Autodesk Inventor part; units mm, degrees
ref_plane "YZ Plane" through (0, 0, 0) normal (1, 0, 0) x (0, 1, 0)
ref_plane "XZ Plane" through (0, 0, 0) normal (0, 1, 0) x (-1, 0, 0)
ref_plane "XY Plane" through (0, 0, 0) normal (0, 0, 1) x (1, 0, 0)
sketch "Sketch1" plane through (0, 0, 0) normal (0, 0, 1) x (1, 0, 0)
  line L0 (-395.4763, 28.0534) -> (214.1237, 28.0534)
  line L1 (214.1237, 28.0534) -> (214.1237, -124.3466)
  line L2 (214.1237, -124.3466) -> (-395.4763, -124.3466)
  line L3 (-395.4763, -124.3466) -> (-395.4763, 28.0534)
  line L4 (100.4888, 124.4295) -> (100.4888, 286.3545)
  line L5 (100.4888, 286.3545) -> (135.4138, 286.3545)
  line L6 (137.9237, 286.3545) -> (137.9237, 124.4295)
  line L7 (137.9237, 124.4295) -> (100.4888, 124.4295)
  point P0 (0, 0)
  dimension "d0" = 609.6
  dimension "d1" = 152.4
  dimension "d7" = 161.925
  dimension "d8" = 34.925
extrude "Extrusion1" add sketch "Sketch1" along normal blind 152.4
sketch "Sketch4" plane through (214.1237, -124.3466, 0) normal (1, 0, 0) x (0, 0, -1)
  circle A0 centre (-76.2, 76.2) radius 5.1594
  line L0 (-152.4, 0) -> (-152.4, 152.4)
  line L1 (0, 152.4) -> (-152.4, 152.4)
  point P0 (0, 124.3466)
  dimension "d1" = 152.4
  dimension "d9" = 10.3187
extrude "Extrusion2" cut sketch "Sketch4" against normal blind 609.6
sketch "Sketch5" plane through (-395.4763, 28.0534, 0) normal (0, 1, 0) x (1, 0, 0)
  line L0 (609.6, -152.4) -> (0, -152.4)
  line L1 (0, -152.4) -> (0, 0)
  line L2 (0, 0) -> (609.6, 0)
  line L3 (609.6, 0) -> (609.6, -152.4)
  line L4 (609.6, -152.4) -> (0, -152.4)
  line L5 (609.6, 0) -> (609.6, -152.4)
  line L6 (0, 0) -> (0, -152.4)
  line L7 (0, 0) -> (609.6, 0)
  line L8 (297.18, -104.775) -> (312.42, -104.775)
  line L9 (312.42, -104.775) -> (312.42, -47.625)
  line L10 (312.42, -47.625) -> (297.18, -47.625)
  line L11 (297.18, -47.625) -> (297.18, -104.775)
  line L12 (297.18, -104.775) -> (312.42, -47.625) construction
  line L13 (312.42, -104.775) -> (297.18, -47.625) construction
  point P0 (395.4763, 0)
  point P1 (297.0135, -78.1466)
  point P2 (312.2535, -78.0634)
  point P3 (312.2535, -74.3366)
  point P4 (304.8, -76.2)
  dimension "d1" = 152.4
  dimension "d48" = 15.24
  dimension "d49" = 57.15
  dimension "d50" = 47.625
  dimension "d51" = 47.625
extrude "Extrusion3" cut sketch "Sketch5" against normal blind 609.6 contours L11 L10 L9 L8
fillet "Fillet1" radius 6.35 4 edges at (-90.6763, 28.0534, 47.625) (-90.6763, 28.0534, 104.775) (-90.6763, -124.3466, 47.625) (-90.6763, -124.3466, 104.775)
chamfer "Chamfer1" distance 3.175 angle 45 1 edges at (214.1237, -48.1466, 81.3594) measured on face at (16.0037, -48.5618, 71.0574)
chamfer "Chamfer2" distance 3.175 angle 45 1 edges at (-395.4763, -48.1466, 81.3594) measured on face at (-296.4163, -48.5618, 71.0574)
sketch "Sketch6" plane through (-395.4763, 28.0534, 0) normal (0, 1, 0) x (1, 0, 0)
  line L0 (609.6, 0) -> (609.6, -152.4)
  line L1 (609.6, -152.4) -> (0, -152.4)
  line L2 (0, -152.4) -> (0, 0)
  line L3 (0, 0) -> (609.6, 0)
  line L4 (609.6, -84.5344) -> (609.6, -67.8656)
  line L5 (609.6, -76.2) -> (625.475, -76.2) construction
  circle A0 centre (593.725, -76.2) radius 3.175
  line L6 (0, 0) -> (0, -152.4)
  circle A1 centre (15.875, -76.2) radius 3.175
  line L7 (297.18, -41.275) -> (312.42, -41.275)
  line L8 (312.42, -111.125) -> (312.42, -41.275)
  line L9 (312.42, -111.125) -> (297.18, -111.125)
  line L10 (297.18, -41.275) -> (297.18, -111.125)
  point P0 (395.4763, 0)
  dimension "d1" = 152.4
  dimension "d30" = 6.35
  dimension "d34" = 6.35
extrude "Extrusion4" cut sketch "Sketch6" against normal blind 101.6 contours A0 | A1
sketch "Sketch7" plane through (-395.4763, 28.0534, 0) normal (0, 1, 0) x (1, 0, 0)
  circle A0 centre (593.725, -76.2) radius 3.175 construction
  circle A1 centre (15.875, -76.2) radius 3.175
  line L0 (609.6, 0) -> (609.6, -152.4) construction
  line L1 (609.6, -152.4) -> (0, -152.4)
  line L2 (0, -152.4) -> (0, 0)
  line L3 (0, 0) -> (609.6, 0)
  line L4 (609.6, -152.4) -> (0, -152.4)
  line L5 (565.15, -152.4) -> (565.15, 0) construction
  line L6 (609.6, 0) -> (609.6, -152.4) construction
  line L7 (297.18, -41.275) -> (312.42, -41.275)
  line L8 (312.42, -111.125) -> (312.42, -41.275)
  line L9 (312.42, -111.125) -> (297.18, -111.125)
  line L10 (297.18, -41.275) -> (297.18, -111.125)
  line L11 (609.6, -76.2) -> (629.3437, -76.2) construction
  line L12 (629.3437, -56.1975) -> (609.6, -56.1975) construction
  line L13 (629.3437, -96.2025) -> (609.6, -96.2025) construction
  line L14 (609.6, -96.2025) -> (529.5756, -96.2025) construction
  line L15 (609.6, -56.1975) -> (531.5543, -56.1975) construction
  circle A2 centre (565.15, -96.2025) radius 3.175
  circle A3 centre (565.15, -56.1975) radius 3.175
  point P0 (395.4763, 0)
  dimension "d1" = 152.4
  dimension "d37" = 44.45
  dimension "d85" = 20.0025
  dimension "d86" = 40.005
  dimension "d87" = 6.35
  dimension "d88" = 6.35
  dimension "d89" = 44.45
extrude "Extrusion5" cut sketch "Sketch7" against normal blind 28.575 contours A2 | A3
sketch "Sketch9" plane through (-395.4763, -124.3466, 0) normal (0, -1, 0) x (1, 0, 0)
  line L0 (609.6, 152.4) -> (609.6, 0)
  line L1 (609.6, 0) -> (0, 0)
  line L2 (0, 0) -> (0, 152.4)
  line L3 (0, 152.4) -> (609.6, 152.4)
  line L4 (312.42, 41.275) -> (297.18, 41.275)
  line L5 (297.18, 111.125) -> (297.18, 41.275)
  line L6 (297.18, 111.125) -> (312.42, 111.125)
  line L7 (312.42, 41.275) -> (312.42, 111.125)
  line L8 (0, 76.2) -> (609.6, 76.2) construction
  circle A0 centre (218.44, 76.2) radius 19.685
  point P0 (395.4763, 0)
  dimension "d1" = 152.4
  dimension "d65" = 39.37
  dimension "d66" = 78.74
  dimension "d69" = 0
extrude "Extrusion8" cut sketch "Sketch9" against normal blind 63.5 contours A0
sketch "Sketch10" plane through (0, 0, 152.4) normal (0, 0, 1) x (1, 0, 0)
  line L0 (214.1237, 28.0534) -> (214.1237, -124.3466)
  line L1 (214.1237, -124.3466) -> (-395.4763, -124.3466)
  line L2 (-395.4763, -124.3466) -> (-395.4763, 28.0534)
  line L3 (-395.4763, 28.0534) -> (214.1237, 28.0534)
  line L4 (-157.3513, -124.3466) -> (-196.7213, -124.3466)
  line L5 (-157.3513, -60.8466) -> (-196.7213, -60.8466)
  line L6 (-157.3513, -124.3466) -> (-196.7213, -124.3466)
  line L7 (-157.3513, -92.075) -> (-196.7213, -92.075)
  line L8 (-177.0363, -92.075) -> (-177.0363, -60.8466)
  point P0 (0, 0)
  dimension "d1" = 152.4
  dimension "d72" = 31.2284
hole "Hole1" at (-177.0363, -92.075, 152.4) direction (0, 0, -1) diameter 3.9624 depth 13.6144 tip angle 118
sketch "Sketch11" plane through (214.1237, -124.3466, 0) normal (1, 0, 0) x (0, 0, -1)
  circle A0 centre (-76.2, 12.7) radius 3.175
  circle A1 centre (-76.2, 42.0133) radius 3.175
  point P0 (0, 124.3466)
  dimension "d1" = 152.4
extrude "Extrusion9" cut sketch "Sketch11" against normal blind 28.575
thread "Thread7"
thread "Thread8"
sketch "Sketch12" plane through (0, 0, 0) normal (0, 0, -1) x (-1, 0, 0)
  line L0 (-214.1237, -124.3466) -> (-214.1237, 28.0534) construction
  line L1 (-214.1237, 28.0534) -> (395.4763, 28.0534) construction
  line L2 (395.4763, 28.0534) -> (395.4763, -124.3466) construction
  line L3 (395.4763, -124.3466) -> (-214.1237, -124.3466) construction
  line L4 (90.6763, 28.0534) -> (90.6763, -124.3466) construction
  line L5 (392.3013, -42.9872) -> (392.3013, -53.306)
  line L6 (-36.3237, -111.6466) -> (90.6763, -111.6466) construction
  line L7 (90.6763, -111.6466) -> (90.6763, 15.3534) construction
  line L8 (90.6763, 15.3534) -> (-36.3237, 15.3534) construction
  line L9 (-36.3237, 15.3534) -> (-36.3237, -111.6466) construction
  line L10 (118.2888, 15.3534) -> (-69.9987, 15.3534) construction
  line L11 (118.2888, -10.0466) -> (-69.9987, -10.0466) construction
  line L12 (65.2763, 28.0534) -> (65.2763, -124.3466) construction
  circle A0 centre (65.2763, -10.0466) radius 4.7625
  circle A1 centre (-10.9237, -10.0466) radius 4.7625
  circle A2 centre (65.2763, -86.2466) radius 4.7625
  circle A3 centre (-10.9237, -86.2466) radius 4.7625
  line L13 (63.0639, -10.0466) -> (251.3514, -10.0466) construction
  line L14 (116.0763, 28.0534) -> (116.0763, -124.3466) construction
  circle A4 centre (116.0763, -10.0466) radius 4.7625
  circle A5 centre (192.2763, -10.0466) radius 4.7625
  circle A6 centre (116.0763, -86.2466) radius 4.7625
  circle A7 centre (192.2763, -86.2466) radius 4.7625
  point P0 (0, 0)
  point P1 (181.3527, 0)
  dimension "d1" = 152.4
  dimension "d97" = 127
  dimension "d98" = 127
  dimension "d99" = 25.4
  dimension "d100" = 25.4
  dimension "d101" = 9.525
  dimension "d104" = 76.2
  dimension "d107" = 76.2
extrude "Extrusion10" cut sketch "Sketch12" against normal through all
properties part number "block"
Work out the finished part from the listing and answer in its coordinate system (mm). A direction names the side the tool comes from. Give positions to 0.01 mm unless a question says otherwise; leave off trailing zeros. Answer as CSV lines item,"result".
Q1. Find the intervals of material crossed by probe 1 along Y at (x, z) = (205.25, 76.2); probe 2 along Y at (x, z) = (-190.5, 98); probe 3 along Y at (x, z) = (198, 76.2), in increasing order. Write a range as [from, to].
A:
probe 1,"y = [-124.35, -114.82], [-108.47, -85.51], [-79.16, -53.31], [-42.99, 28.05]"
probe 2,"y = [-124.35, -90.67], [-81.83, -14.47], [-5.63, 28.05]"
probe 3,"y = [-124.35, -114.82], [-108.47, -85.51], [-79.16, -73.55]"
Q2. A tool of negligible diameter and unlimited length cuts with its end or side. For faces 1 (the conical face through (-392.5, -51.77, 80.15)), 2 (the flat face through (-177, -60.847, 76)), 3 (the flat face through (-91, -47, 104.775)), from which of +Z, -Z, +X, -X, +Y, -Y can it reach the whole face along a straight path? Write none if from no direction.
A:
face 1,"-X"
face 2,"-Y"
face 3,"+Y, -Y"
Q3. The mould has two halves that part along Y. Classify faces 4 (the flat face through (-86, -124.347, 41)), 5 (the cylindrical face through (-243.241, -47.92, 81.354)), 6 (the flat face through (-83.056, -47, 84)): +Y half, -Y half, draft (parallel to the pull), parting line (faces both ways), or undercut.
A:
face 4,"-Y half"
face 5,"undercut"
face 6,"draft"
Q4. Given P1, Ø5, axis at y = -82.33, z = 76.2, coming from the +X side; P2, Ø3, axis at x = -177.04, y = -92.08, coming from the +Z side, each flat-ended and moving along its own axis, determine where each tip first touches the part or whether it passes through.
A:
P1,"stops at x = 185.55"
P2,"stops at z = 138.5"
